from build123d import *

# Parameters (mm, degrees)
SKETCH1_W                 = 32.5
SKETCH1_H                 = 48
BOSS_EXTRUDE1_DEPTH       = 3
F_2_56_TAPPED_HOLE1_D     = 1.778
F_2_56_TAPPED_HOLE1_DEPTH = 7.46583491
F_2_56_TAPPED_HOLE1_TIP   = 0.53416509
F_2_56_TAPPED_HOLE2_D     = 1.778
F_2_56_TAPPED_HOLE2_DEPTH = 7.46583491
F_2_56_TAPPED_HOLE2_TIP   = 0.53416509
F_8_32_TAPPED_HOLE1_D     = 3.4544
F_8_32_TAPPED_HOLE1_DEPTH = 9.672193539
F_8_32_TAPPED_HOLE1_TIP   = 1.037806461
SKETCH16_R                = 1.22
CUT_EXTRUDE4_DEPTH        = 3


with BuildPart() as part:
    # Sketch1 → Boss-Extrude1 (new body)
    with BuildSketch(Plane(origin=(0, 0, 0), x_dir=(1, 0, 0), z_dir=(0, 1, 0))):
        with Locations((16.25, 24)):
            Rectangle(SKETCH1_W, SKETCH1_H)
    extrude(amount=BOSS_EXTRUDE1_DEPTH)

    # #2-56 Tapped Hole1
    with Locations(Plane.ZY):
        with Locations((-36, 1.5), (-12, 1.5)):
            Hole(F_2_56_TAPPED_HOLE1_D / 2, depth=F_2_56_TAPPED_HOLE1_DEPTH)
            with Locations((0, 0, -(F_2_56_TAPPED_HOLE1_DEPTH + F_2_56_TAPPED_HOLE1_TIP / 2))):  # 118° drill point
                Cone(0, F_2_56_TAPPED_HOLE1_D / 2, F_2_56_TAPPED_HOLE1_TIP, mode=Mode.SUBTRACT)

    # #2-56 Tapped Hole2
    with Locations(Plane(origin=(32.5, 0, 0), x_dir=(0, 0, -1), z_dir=(1, 0, 0))):
        with Locations((12, 1.5), (36, 1.5)):
            Hole(F_2_56_TAPPED_HOLE2_D / 2, depth=F_2_56_TAPPED_HOLE2_DEPTH)
            with Locations((0, 0, -(F_2_56_TAPPED_HOLE2_DEPTH + F_2_56_TAPPED_HOLE2_TIP / 2))):  # 118° drill point
                Cone(0, F_2_56_TAPPED_HOLE2_D / 2, F_2_56_TAPPED_HOLE2_TIP, mode=Mode.SUBTRACT)

    # #8-32 Tapped Hole1
    with Locations(Plane(origin=(0, 3, 0), x_dir=(1, 0, 0), z_dir=(0, 1, 0))):
        with Locations((16.25, 19.275)):
            Hole(F_8_32_TAPPED_HOLE1_D / 2, depth=F_8_32_TAPPED_HOLE1_DEPTH)
            with Locations((0, 0, -(F_8_32_TAPPED_HOLE1_DEPTH + F_8_32_TAPPED_HOLE1_TIP / 2))):  # 118° drill point
                Cone(0, F_8_32_TAPPED_HOLE1_D / 2, F_8_32_TAPPED_HOLE1_TIP, mode=Mode.SUBTRACT)

    # Sketch16 → Cut-Extrude4 (cut)
    with BuildSketch(Plane(origin=(0, 3, 0), x_dir=(1, 0, 0), z_dir=(0, 1, 0))):
        with Locations(Location((8.5, 30.48, 0), (0, 0, 270))):
            Circle(SKETCH16_R)
        with Locations(Location((24, 30.48, 0), (0, 0, 270))):
            Circle(SKETCH16_R)
        with Locations(Location((8.5, 8.07, 0), (0, 0, 270))):
            Circle(SKETCH16_R)
        with Locations(Location((24, 8.07, 0), (0, 0, 270))):
            Circle(SKETCH16_R)
    extrude(amount=-CUT_EXTRUDE4_DEPTH, mode=Mode.SUBTRACT)


solid = part.part
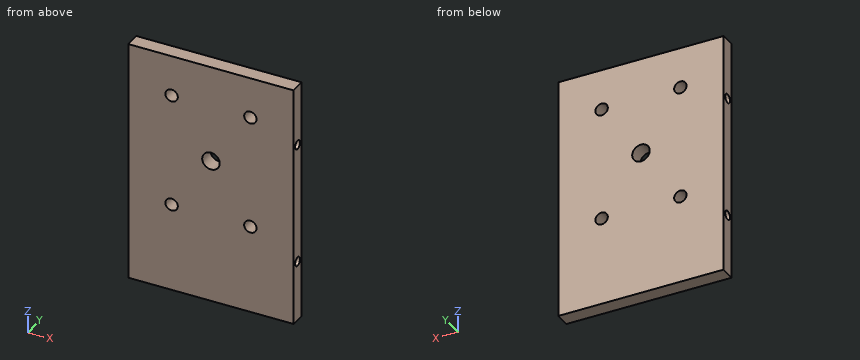
CAD build for the part. Positions are in the model's coordinates, mm. Give positions to 0.01 mm unless a question says otherwise; leave off trailing zeros. Write each loop counter-clockwise with the first axis right and the second up, starting at its lowest first coordinate (ties: lowest second). Pieces come first, ordered by that corner, then holes. Notation, with made-up numbers: (75.5, 14.5) -> (130.5, 14.5) arc R5 ccw to (130.5, 22.5) -> close; hole circle Ø5 at (-39.5, 60.25). An arc over 180 degrees is marked (long way). Return JSON: item names as keys, results as strings.
Item 1: Band-saw the part on A-A (x = 8.5). List the corners of the cut face in (y, z).
Answer below:
{"outline": "(0, -48) -> (3, -48) -> (3, -31.7) -> (0, -31.7) -> close; (0, -29.26) -> (3, -29.26) -> (3, -9.29) -> (0, -9.29) -> close; (0, -6.85) -> (3, -6.85) -> (3, 0) -> (0, 0) -> close"}
Item 2: Drill centre lines: probe 1 along X at (y, z) = (1.05, -30.48); probe 2 along Z at (x, y) = (6.25, 1.5); probe 3 along Z at (x, y) = (5, 1.8). Where is each one in solid material? Low to high.
Answer below:
{"probe 1": "x = 0 to 7.28, 9.72 to 22.78, 25.22 to 32.5", "probe 2": "z = -48 to -36.89, -35.11 to -12.89, -11.11 to 0", "probe 3": "z = -48 to -36.84, -35.16 to -12.84, -11.16 to 0"}
Item 3: Band-saw the part on D-D (x = 29.5). List the corners of the cut face in (y, z).
Answer below:
{"outline": "(0, -48) -> (3, -48) -> (3, 0) -> (0, 0) -> close; hole circle Ø1.78 at (1.5, -36); hole circle Ø1.78 at (1.5, -12)"}
Item 4: Band-saw the part on C-C (x = 16.25). List the corners of the cut face in (y, z), then the cut area to 3 significant figures.
Answer below:
{"outline": "(0, -48) -> (3, -48) -> (3, -21) -> (0, -21) -> close; (0, -17.55) -> (3, -17.55) -> (3, 0) -> (0, 0) -> close", "area": "134 mm2"}
Item 5: Drop flat-ended pins along their axis: pin 1 (1.5 mm diameter, centred on x = 8.5, z = -8.07, fed in from +Y); pin 2 (1.6 mm diameter, centred on y = 1.5, z = -12, fed in from -X). Give the stop position or say it passes through.
Answer below:
{"pin 1": "passes through", "pin 2": "stops at x = 7.52"}
Item 6: Band-saw the part on B-B (z = -8.07). List the corners of the cut face in (x, y), then the cut area to 3 significant figures.
Answer below:
{"outline": "(0, 0) -> (7.28, 0) -> (7.28, 3) -> (0, 3) -> close; (9.72, 0) -> (22.78, 0) -> (22.78, 3) -> (9.72, 3) -> close; (25.22, 0) -> (32.5, 0) -> (32.5, 3) -> (25.22, 3) -> close", "area": "82.9 mm2"}
